Job drawing, mm, ordinate dimensions from the low corner. One solid piece. A direction names the side the tool comes from. Round coordinates to 2 decimals unless told otherwise and drop trailing zeros. Loops run counter-clockwise (first coordinate to the right, second up) from the corner with the lowest first, then second, coordinate; pieces in that order, holes last.
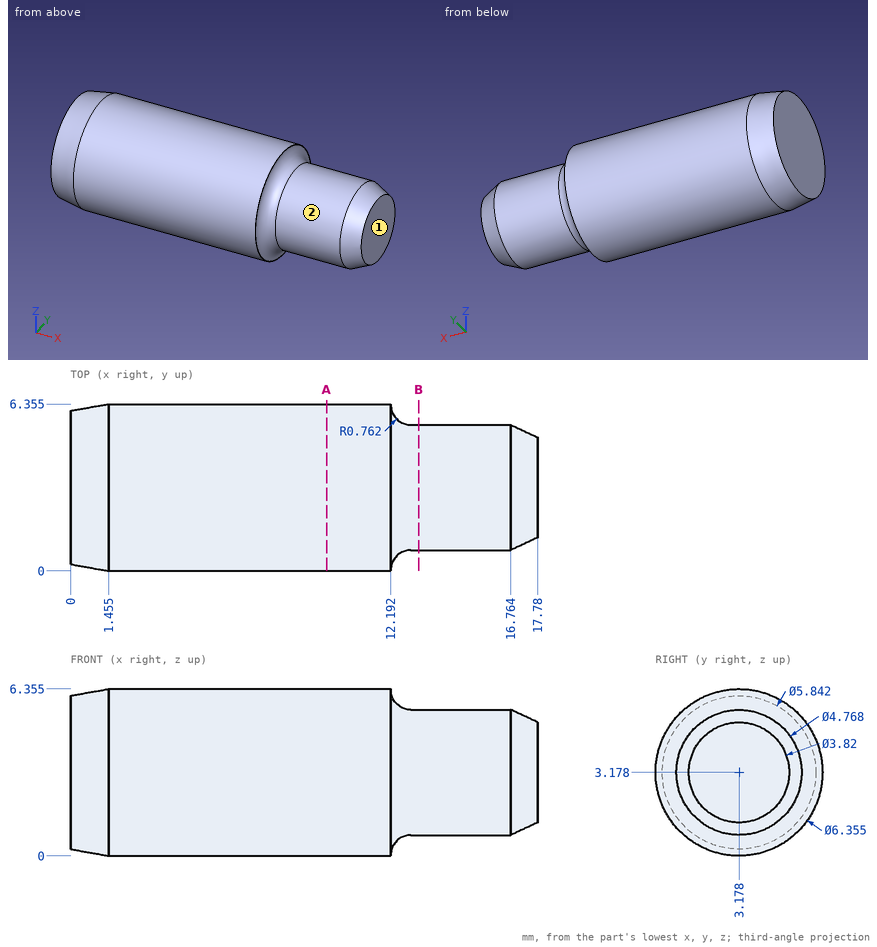
Item 1: Probe line 1 (Z direction, x = 10, y = 3.25) (1 decimal); line 2 (Y direction, x = 5.75, z = 2.75); line 3 (Y direction, x = 14.5, z = 1.5) (1 decimal). List the from-to ranges inside material, lowest first.
Answers follow:
line 1: z = 0 to 6.4
line 2: y = 0.03 to 6.33
line 3: y = 1.5 to 4.9
Item 2: Cut at A-A, the plane x = 9.75. Give the cut face in (y, z) (1 decimal), plus the area to 3 significant figures.
Answers follow:
outline: circle Ø6.4 at (3.2, 3.2)
area: 31.7 mm2
Item 3: Cut at B-B, the plane x = 13.25. Give the cut face in (y, z).
Answers follow:
outline: circle Ø4.77 at (3.18, 3.18)
Item 4: 3-axis set-ups, long thin cutter, end or side, ignore diameter. For the marked faces 1 and 2: which of +Z, -Z, +X, -X, +Y, -Y reach the whole face in a straight line?
Answers follow:
face 1: +Z, -Z, +X, +Y, -Y
face 2: +X
Item 5: Flat gauge pins, fed straight in: P1, Ø1, axis at x = 14.5, y = 3.5, coming from the +Z side; P2, Ø1.5, axis at x = 12, z = 1.5, coming from the -Y side; P3, Ø1, axis at x = 2, z = 5, coming from the -Y side. Where does each tip first touch, or does it go through?
Answers follow:
P1: stops at z = 5.56
P2: stops at y = 0.14
P3: stops at y = 0.29
